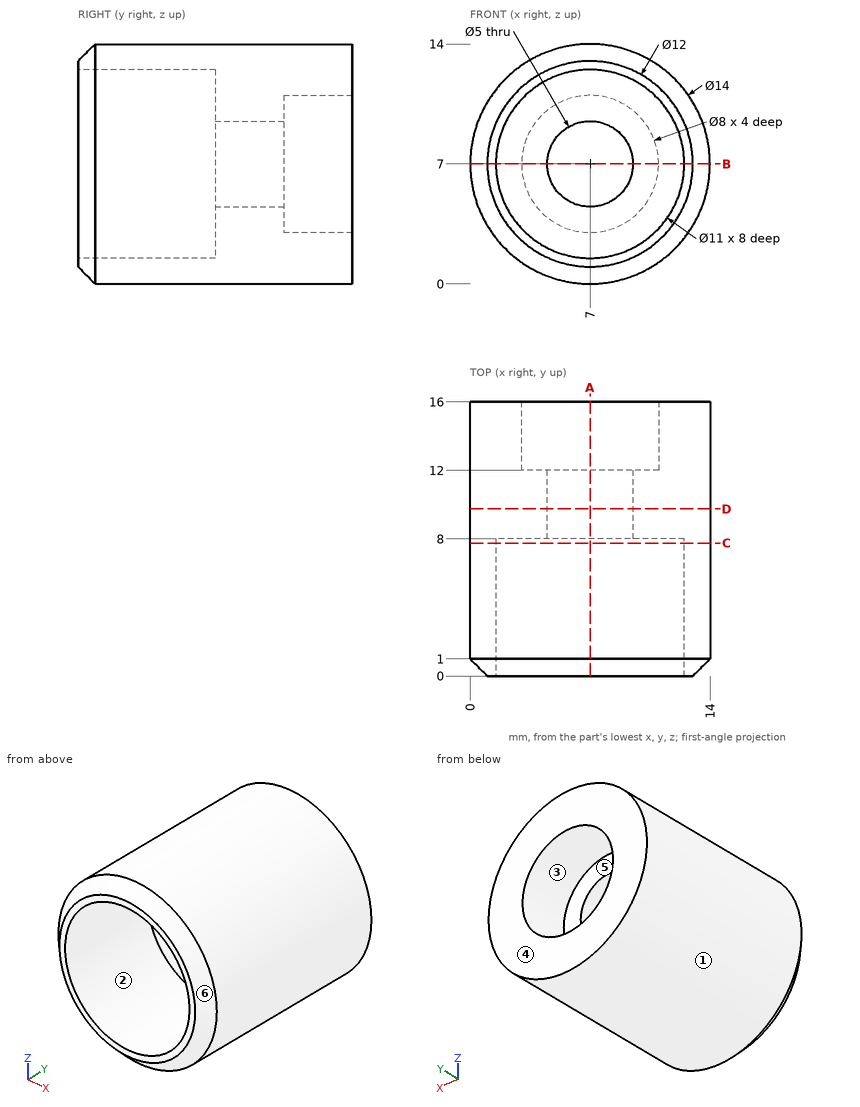
Source: three-view drawing plus pictorial views. Frame: mm from the lowest corner of the part. A direction names the side the tool comes from. Round coordinates to 2 decimals unless told otherwise and drop trailing zeros. Order: outer loops, then holes, each group sorted by start corner. A loop starts at its lowest first (then second) coordinate and runs counter-clockwise, first axis right, second up. Notation, with made-up numbers: (-18.75, 39.5) -> (7.25, 39.5) arc R27 cw to (7.25, 76.5) -> close; hole circle Ø5 at (-35.75, -20). An arc over 180 degrees is marked (long way). Use one line per item in the form item = value.
(1) Section A-A on x = 7. Return loops of the section in (y, z), and give its area (3 significant figures).
Results list:
outline = (0, 1) -> (1, 0) -> (16, 0) -> (16, 3) -> (12, 3) -> (12, 4.5) -> (8, 4.5) -> (8, 1.5) -> (0, 1.5) -> close; (0, 12.5) -> (8, 12.5) -> (8, 9.5) -> (12, 9.5) -> (12, 11) -> (16, 11) -> (16, 14) -> (1, 14) -> (0, 13) -> close
area = 83.0 mm^2
(2) Section D-D on y = 9.75. Return loops of the section in (x, z).
Results list:
outline = circle Ø14 at (7, 7); hole circle Ø5 at (7, 7)
(3) Section B-B on z = 7. Return loops of the section in (x, y).
Results list:
outline = (0, 1) -> (1, 0) -> (1.5, 0) -> (1.5, 8) -> (4.5, 8) -> (4.5, 12) -> (3, 12) -> (3, 16) -> (0, 16) -> close; (9.5, 8) -> (12.5, 8) -> (12.5, 0) -> (13, 0) -> (14, 1) -> (14, 16) -> (11, 16) -> (11, 12) -> (9.5, 12) -> close
(4) Section C-C on y = 7.75. Return loops of the section in (x, z), and give its area (3 significant figures).
Results list:
outline = circle Ø14 at (7, 7); hole circle Ø11 at (7, 7)
area = 58.9 mm^2
(5) Draft query along X for the marked faces 1, 2, 3 and 4. Return one class per face: pulls with the +X half, pulls with the -X half, needs draft (parallel to the pull), parting line crosses it, or undercut.
Results list:
face_1 = parting line crosses it
face_2 = undercut
face_3 = undercut
face_4 = needs draft
(6) Access query for the marked faces 5 and 6. Directions: +Z, -Z, +X, -X, +Y, -Y. A direction counts if a zero-diameter tool reaches every point of the face in a straight line with its end or side. Return the directions, or none.
Results list:
face_5 = +Y
face_6 = -Y
(7) Ray query, probe 1 along Z at (x, y) = (7, 15.1); probe 2 along Z at (x, y) = (7, 9.65); probe 3 along Y at (x, z) = (5.75, 11.75). Return the intervals inside material, ascending. Write a range as [from, to].
Results list:
probe_1 = [0, 3], [11, 14]
probe_2 = [0, 4.5], [9.5, 14]
probe_3 = [8, 16]
(8) First-contact query: pin 1 Ø1 at (y, z) = (12.5, 10.5) entering from -X; pin 2 Ø1 at (x, y) = (12, 8) entering from +Z; pin 3 Ø4 at (x, y) = (2.5, 7.5) entering from -Z; pin 4 Ø4 at (x, z) = (7, 7) entering from -Y. Flat tips, straight axial feed; report the tip coordinate or a pass-through.
Results list:
pin_1 = 0.68
pin_2 = 12.36
pin_3 = 0.46
pin_4 = through
